The model under review builds one solid part; all positions refer to its coordinate system, in mm. A direction names the side the tool comes from. Round coordinates to 2 decimals unless told otherwise and drop trailing zeros. Loops run counter-clockwise (first coordinate to the right, second up) from the corner with the lowest first, then second, coordinate; pieces in that order, holes last. Notation, with made-up numbers: M -9.75,52 L 37.25,52 A23 cw 37.25,87 Z; hole C 79.25,85 d4. An arc over 180 degrees is marked long. Return JSON: item names as keys, results as strings. Group by question number.
Q1. Consider section A-A (x = -32). State the section outline as (y, z) points, and give its area (4 significant figures).
Q2. Clearance check with flat-ended pins moving along their axes: pin 1 Ø2 at (y, z) = (-25, 4.5) entering from -X; pin 2 Ø1.3 at (y, z) = (60.5, 2) entering from +X; pin 3 Ø1.5 at (y, z) = (47, 3) entering from +X. State where each tip first meets the part, or that it passes through.
Q3. Draft analysis for pull direction X (two halves, no side actions). For faces 5 (the face through (-45, 100, 3)), 6 (the face through (115, 47, 3)), 7 (the face through (-115, 47, 3)), state which applies: pulls with the +X half, pulls with the -X half, needs draft (parallel to the pull), parting line crosses it, or undercut.
Q4. Consider section B-B (z = 1.7). Count the separate pieces of the cut face and the enclosed holes in it, and give its area (3 significant figures).
Q5. For faces 1 (the face through (117, 61.46, 3)), 2 (the face through (14, 105, 2)), 3 (the face through (-81, 105, 2)), 4 (the face through (-118, 61.46, 3)), list the 3-axis set-ups (+Z, -Z, +X, -X, +Y, -Y) from which the entire face can be reached by the end or side of a thin tool; tool diameter is ignored.
Q6. To check wall thickness, follow line 1 along Y through (x, z) = (-13, 2.9); line 2 along X through (y, z) = (9.5, 1.55); line 3 along Y through (x, z) = (107.5, 2.2). State the ranges of each line that lie inside material, in increasing order.
from build123d import *

# Parameters (mm, degrees)
BOSS_EXTRUDE1_DEPTH = 5
CUT_EXTRUDE1_DEPTH  = 5
CUT_EXTRUDE4_DEPTH  = 5
BOSS_EXTRUDE3_DEPTH = 5
SKETCH8_R           = 2.1
SKETCH8_W           = 5
SKETCH8_H           = 10
SKETCH8_W_2         = 40
SKETCH8_H_2         = 5
CUT_EXTRUDE5_DEPTH  = 10
BOSS_EXTRUDE4_DEPTH = 5
SKETCH10_W          = 77.5
SKETCH10_H          = 80
BOSS_EXTRUDE5_DEPTH = 5
CUT_EXTRUDE6_DEPTH  = 5
SKETCH12_R          = 2.1
SKETCH12_W          = 5
SKETCH12_H          = 35
CUT_EXTRUDE7_DEPTH  = 5
BOSS_EXTRUDE6_DEPTH = 5
SKETCH14_W          = 5
SKETCH14_H          = 10.4
SKETCH14_H_2        = 35.4
SKETCH14_W_2        = 40.4
SKETCH14_H_3        = 5
CUT_EXTRUDE8_DEPTH  = 10


with BuildPart() as part:
    # Sketch1 → Boss-Extrude1 (new body)
    with BuildSketch(Plane.XY):
        Polygon((-120, 40), (-42.5, 40), (-42.5, -40), (-120, -40), (-120, -105), (120, -105), (120, -40), (42.5, -40), (42.5, 40), (120, 40), (120, 105), (-120, 105), align=None)
    extrude(amount=BOSS_EXTRUDE1_DEPTH)

    # Sketch2 → Cut-Extrude1 (cut)
    with BuildSketch(Plane.XY.offset(5)):
        Polygon((40, -55.717967697), (-40, -55.717967697), (-80, -125), (-40, -194.282032303), (40, -194.282032303), (80, -125), align=None)
    extrude(amount=-CUT_EXTRUDE1_DEPTH, mode=Mode.SUBTRACT)

    # Sketch5 → Cut-Extrude4 (cut)
    with BuildSketch(Plane.XY.offset(5)):
        Polygon((-97.823933369, 105), (-120, 73.319904814), (-120, 105), align=None)
        Polygon((97.823933369, 105), (120, 105), (120, 73.319904814), align=None)
    extrude(amount=-CUT_EXTRUDE4_DEPTH, mode=Mode.SUBTRACT)

    # Sketch7 → Boss-Extrude3 (add)
    with BuildSketch(Plane(origin=(0, 0, 0), x_dir=(-1, 0, 0), z_dir=(0, 0, -1))):
        Polygon((120, -40), (120, -105), (89.53, -105), (111.53, -122.5), (129.53, -122.5), (129.53, -40), align=None)
    boss_extrude3 = extrude(amount=-BOSS_EXTRUDE3_DEPTH)

    # Mirror2: Boss-Extrude3 across plane
    add(boss_extrude3.mirror(Plane(origin=(0, 0, 0), x_dir=(0, 0, 1), z_dir=(1, 0, 0))))

    # Sketch8 → Cut-Extrude5 (cut)
    with BuildSketch(Plane.XY.offset(5)):
        with Locations((0, 102.5)):
            Circle(SKETCH8_R)
        with Locations((106.863886883, 87.726296546)):
            Circle(SKETCH8_R)
        with Locations((117.5, 56.659952407)):
            Circle(SKETCH8_R)
        with Locations(Location((-117.5, 56.659952407, 0), (0, 0, 180))):
            Circle(SKETCH8_R)
        with Locations(Location((-106.863886883, 87.726296546, 0), (0, 0, 180))):
            Circle(SKETCH8_R)
        Polygon((-113.212934267, 83.015713003), (-116.080245989, 78.9195534), (-111.984086387, 76.052241679), (-109.116774665, 80.148401281), align=None)
        Polygon((-100.514839499, 92.436880089), (-104.610999102, 95.304191811), (-101.74368738, 99.400351413), (-97.647527778, 96.533039691), align=None)
        with Locations((-117.5, 46.659952407)):
            Rectangle(SKETCH8_W, SKETCH8_H)
        with Locations((-117.5, 66.659952407)):
            Rectangle(SKETCH8_W, SKETCH8_H)
        with Locations((-45, 102.5)):
            Rectangle(SKETCH8_W_2, SKETCH8_H_2)
        with Locations((45, 102.5)):
            Rectangle(SKETCH8_W_2, SKETCH8_H_2)
        with Locations((117.5, 66.659952407)):
            Rectangle(SKETCH8_W, SKETCH8_H)
        with Locations((117.5, 46.659952407)):
            Rectangle(SKETCH8_W, SKETCH8_H)
        Polygon((104.610999102, 95.304191811), (101.74368738, 99.400351413), (97.647527778, 96.533039691), (100.514839499, 92.436880089), align=None)
        Polygon((109.116774665, 80.148401281), (113.212934267, 83.015713003), (116.080245989, 78.9195534), (111.984086387, 76.052241679), align=None)
    extrude(amount=-CUT_EXTRUDE5_DEPTH, mode=Mode.SUBTRACT)

    # Sketch9 → Boss-Extrude4 (add)
    with BuildSketch(Plane.XY.offset(5)):
        with BuildLine():
            Line((-3.122498999, 105), (3.122498999, 105))
            ThreePointArc((3.122498999, 105), (0, 106.5), (-3.122498999, 105))
        make_face()
        with BuildLine():
            Line((107.121331088, 91.718003259), (110.702602281, 86.601901555))
            ThreePointArc((110.702602281, 86.601901555), (110.140814565, 90.020145923), (107.121331088, 91.718003259))
        make_face()
        with BuildLine():
            Line((120, 59.782451406), (120, 53.537453408))
            ThreePointArc((120, 53.537453408), (121.5, 56.659952407), (120, 59.782451406))
        make_face()
        with BuildLine():
            Line((-120, 59.782451406), (-120, 53.537453408))
            ThreePointArc((-120, 53.537453408), (-121.5, 56.659952407), (-120, 59.782451406))
        make_face()
        with BuildLine():
            Line((-107.121331088, 91.718003259), (-110.702602281, 86.601901555))
            ThreePointArc((-110.702602281, 86.601901555), (-110.140814565, 90.020145923), (-107.121331088, 91.718003259))
        make_face()
    extrude(amount=-BOSS_EXTRUDE4_DEPTH)

    # Sketch10 → Boss-Extrude5 (add)
    with BuildSketch(Plane.XY.offset(5)):
        with Locations((-81.25, 0)):
            Rectangle(SKETCH10_W, SKETCH10_H)
        Polygon((-68.452994616, -105), (68.452994616, -105), (40, -55.717967697), (-40, -55.717967697), align=None)
        with Locations((81.25, 0)):
            Rectangle(SKETCH10_W, SKETCH10_H)
    extrude(amount=-BOSS_EXTRUDE5_DEPTH)

    # Sketch11 → Cut-Extrude6 (cut)
    with BuildSketch(Plane.XY.offset(5)):
        Polygon((-120, -40), (-120, -105), (120, -105), (120, -40), (129.53, -40), (129.53, -122.5), (-129.53, -122.5), (-129.53, -40), align=None)
    extrude(amount=-CUT_EXTRUDE6_DEPTH, mode=Mode.SUBTRACT)

    # Sketch12 → Cut-Extrude7 (cut)
    with BuildSketch(Plane.XY.offset(5)):
        with Locations((-117.5, 29.159952407)):
            Circle(SKETCH12_R)
        with Locations((-117.5, -30.840047593)):
            Circle(SKETCH12_R)
        with Locations(Location((117.5, -30.840047593, 0), (0, 0, 180))):
            Circle(SKETCH12_R)
        with Locations(Location((117.5, 29.159952407, 0), (0, 0, 180))):
            Circle(SKETCH12_R)
        with Locations((-117.5, -0.840047593)):
            Rectangle(SKETCH12_W, SKETCH12_H)
        with Locations((117.5, -0.840047593)):
            Rectangle(SKETCH12_W, SKETCH12_H)
    extrude(amount=-CUT_EXTRUDE7_DEPTH, mode=Mode.SUBTRACT)

    # Sketch13 → Boss-Extrude6 (add)
    with BuildSketch(Plane.XY.offset(5)):
        with BuildLine():
            Line((-120, 32.282451406), (-120, 26.037453408))
            ThreePointArc((-120, 26.037453408), (-121.5, 29.159952407), (-120, 32.282451406))
        make_face()
        with BuildLine():
            Line((-120, -27.717548594), (-120, -33.962546592))
            ThreePointArc((-120, -33.962546592), (-121.5, -30.840047593), (-120, -27.717548594))
        make_face()
        with BuildLine():
            Line((120, -27.717548594), (120, -33.962546592))
            ThreePointArc((120, -33.962546592), (121.5, -30.840047593), (120, -27.717548594))
        make_face()
        with BuildLine():
            Line((120, 32.282451406), (120, 26.037453408))
            ThreePointArc((120, 26.037453408), (121.5, 29.159952407), (120, 32.282451406))
        make_face()
    extrude(amount=-BOSS_EXTRUDE6_DEPTH)

    # Sketch14 → Cut-Extrude8 (cut)
    with BuildSketch(Plane.XY.offset(5)):
        Polygon((-104.725691571, 95.140345427), (-100.629531968, 92.273033705), (-97.532835309, 96.696886076), (-101.628994911, 99.564197797), align=None)
        Polygon((-112.098778856, 75.888395294), (-116.194938458, 78.755707016), (-113.098241799, 83.179559387), (-109.002082196, 80.312247665), align=None)
        with Locations((-117.5, 66.659952407)):
            Rectangle(SKETCH14_W, SKETCH14_H)
        with Locations((-117.5, 46.659952407)):
            Rectangle(SKETCH14_W, SKETCH14_H)
        with Locations((-117.5, -0.840047593)):
            Rectangle(SKETCH14_W, SKETCH14_H_2)
        with Locations((-45, 102.5)):
            Rectangle(SKETCH14_W_2, SKETCH14_H_3)
        with Locations((45, 102.5)):
            Rectangle(SKETCH14_W_2, SKETCH14_H_3)
        with Locations((117.5, -0.840047593)):
            Rectangle(SKETCH14_W, SKETCH14_H_2)
        with Locations((117.5, 46.659952407)):
            Rectangle(SKETCH14_W, SKETCH14_H)
        with Locations((117.5, 66.659952407)):
            Rectangle(SKETCH14_W, SKETCH14_H)
        Polygon((113.098241799, 83.179559387), (109.002082196, 80.312247665), (112.098778856, 75.888395294), (116.194938458, 78.755707016), align=None)
        Polygon((97.532835309, 96.696886076), (101.628994911, 99.564197797), (104.725691571, 95.140345427), (100.629531968, 92.273033705), align=None)
    extrude(amount=-CUT_EXTRUDE8_DEPTH, mode=Mode.SUBTRACT)


solid = part.part
Values:
{
 "1": {"outline": "M -105,0 L 100,0 L 100,5 L -105,5 Z", "area": "1,025 mm2"},
 "2": {"pin 1": "stops at x = -120", "pin 2": "stops at x = 120", "pin 3": "stops at x = 115"},
 "3": {"face 5": "undercut", "face 6": "pulls with the +X half", "face 7": "pulls with the -X half"},
 "4": {"separate pieces": "1", "enclosed holes": "9", "area": "48,600 mm2"},
 "5": {"face 1": "+Z, -Z, +X", "face 2": "+Z, -Z, +X, +Y", "face 3": "+Z, -Z, -X, +Y", "face 4": "+Z, -Z, -X"},
 "6": {"line 1": "y = -105 to 105", "line 2": "x = -115 to 115", "line 3": "y = -105 to 85.72, 89.73 to 91.68"}
}
